Job drawing, mm, ordinate dimensions from the low corner. One solid piece. Round coordinates to 2 decimals unless told otherwise and drop trailing zeros. Loops run counter-clockwise (first coordinate to the right, second up) from the corner with the lowest first, then second, coordinate; pieces in that order, holes last.
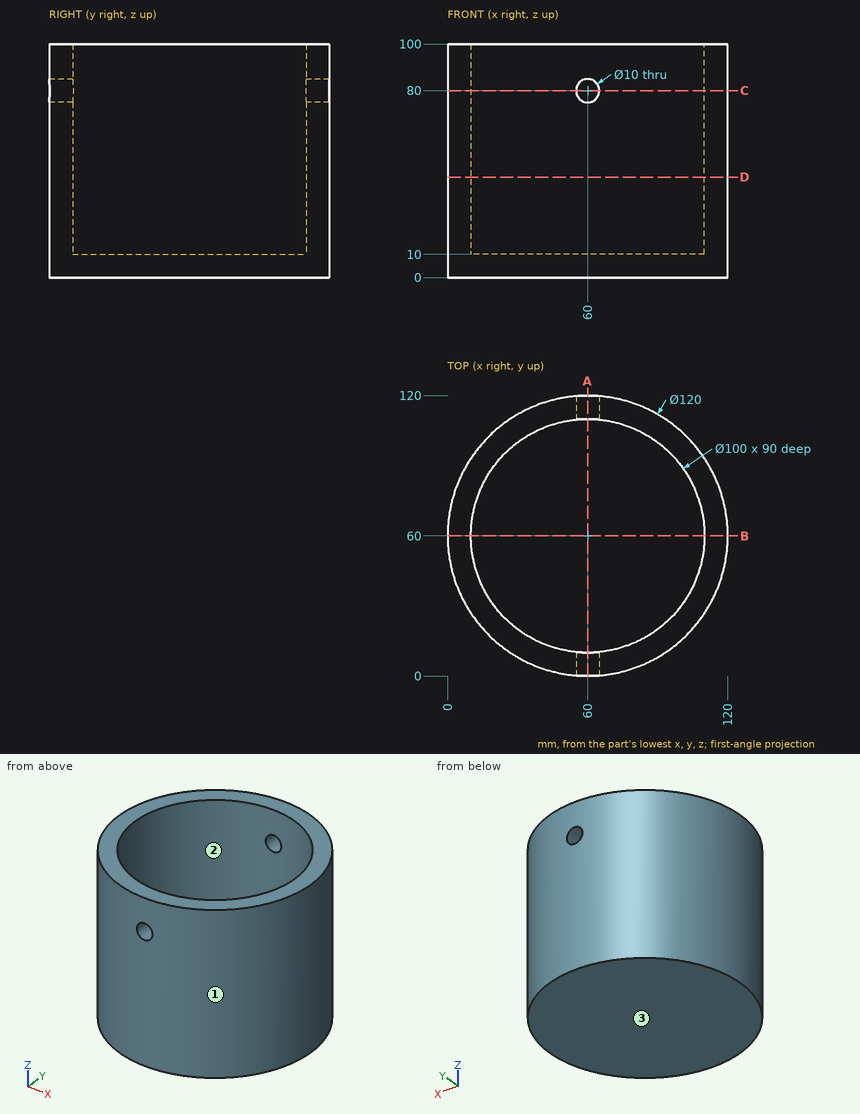
1) Slice it at D-D, the plane z = 43. Give the cut face in (x, y), then the cut area to 3 significant figures.
Values:
outline: circle Ø120 at (60, 60); hole circle Ø100 at (60, 60)
area: 3,460 mm2
2) Slice it at B-B, the plane y = 60. Give the cut face in (x, z).
Values:
outline: (0, 0) - (120, 0) - (120, 100) - (110, 100) - (110, 10) - (10, 10) - (10, 100) - (0, 100) - close
3) Wall check: line 1 along Y through (x, z) = (60, 57.5); line 2 along Z through (x, y) = (87.5, 57); line 3 along X through (y, z) = (43.5, 65). Give the ranges that are in metal, low to high.
Values:
line 1: y = 0 to 10, 110 to 120
line 2: z = 0 to 10
line 3: x = 2.31 to 12.8, 107.2 to 117.69
4) Slice it at A-A, the plane x = 60. Give the cut face in (y, z).
Values:
outline: (0, 0) - (120, 0) - (120, 75) - (110, 75) - (110, 10) - (10, 10) - (10, 75) - (0, 75) - close; (0, 85) - (10, 85) - (10, 100) - (0, 100) - close; (110, 85) - (120, 85) - (120, 100) - (110, 100) - close
5) Mould opens along X. For the marked faces 1, 2 and 3 say: released by +X, released by -X, zero draft, split by the parting line, or undercut.
Values:
face 1: split by the parting line
face 2: undercut
face 3: zero draft
6) Slice it at C-C, the plane z = 80. Give the cut face in (x, y).
Values:
outline: (55, 0.21) - (55, 10.25) arc R50 cw to (55, 109.75) - (55, 119.79) arc R60 ccw to start; (65, 0.21) arc R60 ccw to (65, 119.79) - (65, 109.75) arc R50 cw to (65, 10.25) - close
7) Drop flat-ended pins along their axis: pin 1 Ø8 at (x, z) = (60, 80) entering from -Y; pin 2 Ø6 at (y, z) = (19, 83) entering from -X; pin 3 Ø3 at (x, z) = (89.5, 70) entering from -Y; pin 4 Ø16 at (x, z) = (60, 80) entering from -Y. Give the stop position or say it passes through.
Values:
pin 1: passes through
pin 2: stops at x = 13.57
pin 3: stops at y = 6.93
pin 4: stops at y = 0
